For this review, use the dimensioned drawing (mm, ordinates from the lowest corner) and the shaded views. Round coordinates to 2 decimals unless told otherwise and drop trailing zeros. Order: outer loops, then holes, each group sorted by start corner. A loop starts at its lowest first (then second) coordinate and runs counter-clockwise, first axis right, second up. Notation, with made-up numbers: (8, -7) -> (67, -7) arc R10 ccw to (67, -1) -> close; hole circle Ø8 at (62.25, 1). An arc over 180 degrees is marked (long way). Use a Markdown table: item, result. Add a question column.
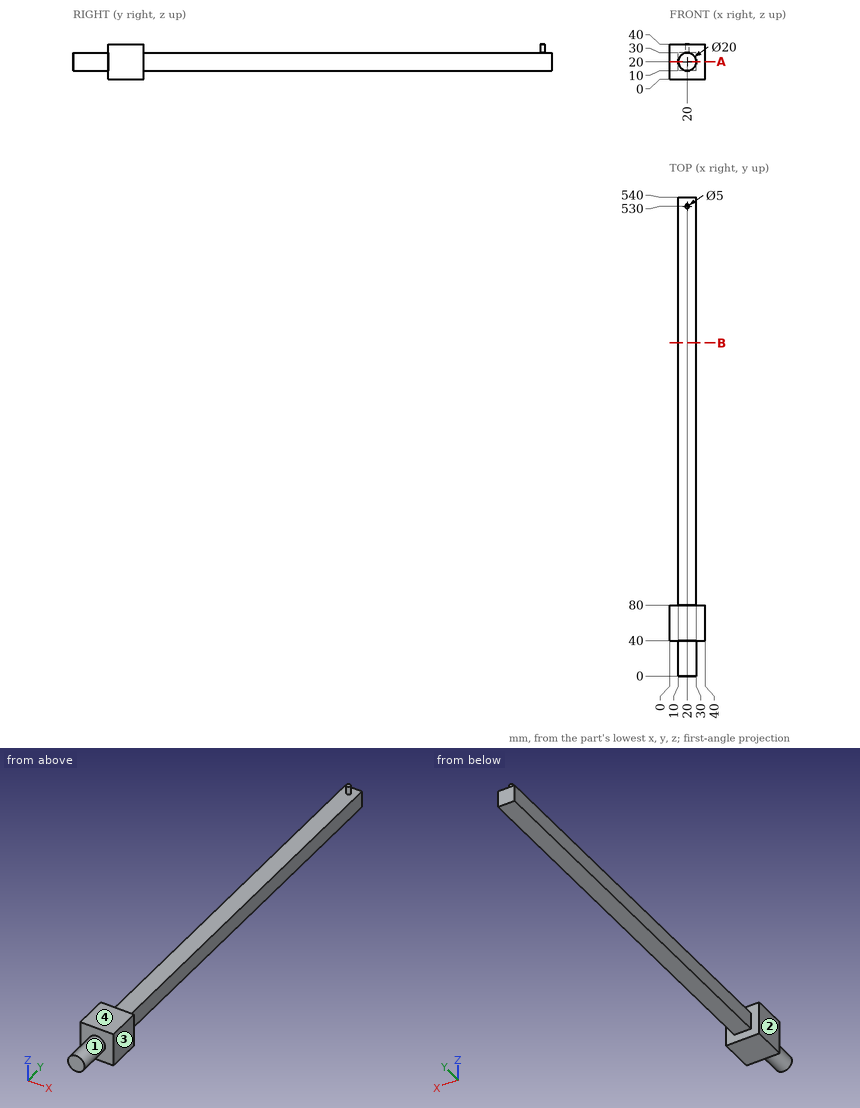
Q1. Wall thickness on line 1 (Z direction, x = 22, y = 133); line 2 (Y direction, x = 33, z = 36): over which ranges is each line inside the solid? List them lowest first. Write a range as [from, to].
Q2. Insertion check: pin 1 (8 mm diameter, centred on y = 299, z = 17.5, fed in from -X); pin 2 (12 mm diameter, centred on x = 27, y = 183.5, fed in from +Z); pin 3 (5 mm diameter, centred on x = 5.5, z = 7, fed in from -Y); pin 4 (12 mm diameter, centred on x = 33.5, y = 81.5, fed in from -Z). Each pin has a flat end and moves straight along its axis. Give the tip position at first contact, or say it passes through.
Q3. Mouldability with a two-part tool opening along X and no side actions: class the marked faces 1, 2, 3 and 4 as pulls with the +X half, pulls with the -X half, needs draft (parallel to the pull), parting line crosses it, or undercut.
Q4. Add section A-A (z = 20). Write out the cut boundary in (x, y), then the cut area to 3 significant figures.
Q5. Add section B-B (y = 376). Write out the cut boundary in (x, z), then the cut area to 3 significant figures.
Report:
| question | item | result |
|---|---|---|
| 1 | line 1 | z = [10, 30] |
| 1 | line 2 | y = [40, 80] |
| 2 | pin 1 | stops at x = 10 |
| 2 | pin 2 | stops at z = 30 |
| 2 | pin 3 | stops at y = 40 |
| 2 | pin 4 | stops at z = 0 |
| 3 | face 1 | parting line crosses it |
| 3 | face 2 | pulls with the -X half |
| 3 | face 3 | pulls with the +X half |
| 3 | face 4 | needs draft |
| 4 | outline | (0, 40) -> (10, 40) -> (10, 0) -> (30, 0) -> (30, 40) -> (40, 40) -> (40, 80) -> (30, 80) -> (30, 540) -> (10, 540) -> (10, 80) -> (0, 80) -> close |
| 4 | area | 11,600 mm² |
| 5 | outline | (10, 10) -> (30, 10) -> (30, 30) -> (10, 30) -> close |
| 5 | area | 400 mm² |
